Can you work these out from the model? Positions are in its coordinate system, mm. Give positions to 0.01 mm unless a question says otherwise; leave off trailing zeros. Order: outer loops, then holes, each group sorted by start corner. A loop starts at its lowest first (then second) coordinate and runs counter-clockwise, first axis right, second up. Notation, with made-up numbers: (-20, 65.5) - (1, 65.5) arc R13 ccw to (1, 72.5) - close; hole circle Ø7 at (7.5, 81). An arc over 180 degrees is marked (long way). Answer as CSV lines item,"result".
```python
from build123d import *

# Parameters (mm, degrees)
SKETCH_1_R      = 1.5
EXTRUDE_1_DEPTH = 27.75


with BuildPart() as part:
    # Эскиз1 → Бобышка-Вытянуть1 (new body)
    with BuildSketch(Plane.XY):
        with BuildLine():
            Line((3.75277675, 0.5), (2.309401077, 3))
            ThreePointArc((2.309401077, 3), (1.943375673, 3.366025404), (1.443375673, 3.5))
            Line((1.443375673, 3.5), (-1.443375673, 3.5))
            ThreePointArc((-1.443375673, 3.5), (-1.943375673, 3.366025404), (-2.309401077, 3))
            Line((-2.309401077, 3), (-3.75277675, 0.5))
            ThreePointArc((-3.75277675, 0.5), (-3.886751346, 0), (-3.75277675, -0.5))
            Line((-3.75277675, -0.5), (-2.309401077, -3))
            ThreePointArc((-2.309401077, -3), (-1.943375673, -3.366025404), (-1.443375673, -3.5))
            Line((-1.443375673, -3.5), (1.443375673, -3.5))
            ThreePointArc((1.443375673, -3.5), (1.943375673, -3.366025404), (2.309401077, -3))
            Line((2.309401077, -3), (3.75277675, -0.5))
            ThreePointArc((3.75277675, -0.5), (3.886751346, 0), (3.75277675, 0.5))
        make_face()
        Circle(SKETCH_1_R, mode=Mode.SUBTRACT)
    extrude(amount=EXTRUDE_1_DEPTH)


solid = part.part
```
1) I want a section at A-A on y = 0. Write out the boundary of the cut face in (x, z).
Answer block:
outline,"(-3.89, 0) - (-1.5, 0) - (-1.5, 27.75) - (-3.89, 27.75) - close; (1.5, 0) - (3.89, 0) - (3.89, 27.75) - (1.5, 27.75) - close"
2) If we mould it in two halves opening along X, with no side actions, what happens to faces 1 (the flat face through (-3, 1.8, 13.7)), 2 (the flat face through (3, -1.8, 13.7)), 3 (the cylindrical face through (-1.5, 0.07, 13.68)), 4 (the flat face through (0, 3.5, 14))? For each: +X half, -X half, draft (parallel to the pull), parting line (faces both ways), or undercut.
Answer block:
face 1,"-X half"
face 2,"+X half"
face 3,"undercut"
face 4,"draft"
3) I want a section at B-B on z = 14. Write out the boundary of the cut face in (x, y).
Answer block:
outline,"(-3.75, -0.5) - (-2.31, -3) arc R1 ccw to (-1.44, -3.5) - (1.44, -3.5) arc R1 ccw to (2.31, -3) - (3.75, -0.5) arc R1 ccw to (3.75, 0.5) - (2.31, 3) arc R1 ccw to (1.44, 3.5) - (-1.44, 3.5) arc R1 ccw to (-2.31, 3) - (-3.75, 0.5) arc R1 ccw to start; hole circle Ø3 at (0, 0)"
4) I need wall thicknesses on line 1 along Y through (x, z) = (0, 21); line 2 along Y through (x, z) = (-0.5, 14.25); line 3 along X through (y, z) = (-1, 5.75). Which ranges of each line are inside material? Lowest first, please. Write a range as [from, to].
Answer block:
line 1,"[-3.5, -1.5], [1.5, 3.5]"
line 2,"[-3.5, -1.41], [1.41, 3.5]"
line 3,"[-3.46, -1.12], [1.12, 3.46]"
5) I'm going to push flat-ended pins straight in: P1, Ø4, axis at y = -2, z = 23.5, coming from the +X side; P2, Ø1.5, axis at x = 3, z = 25, coming from the +Y side; P3, Ø3, axis at y = -2.5, z = 6.5, coming from the -X side. Where does each tip first touch, or does it pass through?
Answer block:
P1,"x = 3.89"
P2,"y = 3.09"
P3,"x = -3.46"
6) I want a section at C-C on x = 0. Write out the boundary of the cut face in (y, z), plus the area to 3 significant figures.
Answer block:
outline,"(-3.5, 0) - (-1.5, 0) - (-1.5, 27.75) - (-3.5, 27.75) - close; (1.5, 0) - (3.5, 0) - (3.5, 27.75) - (1.5, 27.75) - close"
area,"111 mm2"
7) I want a section at D-D on y = 2.75. Write out the boundary of the cut face in (x, z).
Answer block:
outline,"(-2.45, 0) - (2.45, 0) - (2.45, 27.75) - (-2.45, 27.75) - close"
